Design review of the part built by this model. Coordinates are the model's own, in mm. A direction names the side the tool comes from. Give positions to 0.01 mm unless a question says otherwise; leave off trailing zeros. Loops run counter-clockwise (first coordinate to the right, second up) from the corner with the lowest first, then second, coordinate; pieces in that order, holes last.
from build123d import *

# Parameters (mm, degrees)
PAD002_DEPTH    = 10
SKETCH005_R     = 1.5
SKETCH005_W     = 170
SKETCH005_H     = 57.5
POCKET002_DEPTH = 11
PAD003_DEPTH    = 10
PAD004_DEPTH    = 10
POCKET003_DEPTH = 3
SKETCH009_W     = 103.713421
SKETCH009_H     = 5
POCKET004_DEPTH = 10
SKETCH010_W     = 109.037471
SKETCH010_H     = 5
POCKET005_DEPTH = 10
SKETCH011_R     = 1.5
POCKET006_DEPTH = 5
SKETCH012_R     = 3
POCKET007_DEPTH = 3


with BuildPart() as part:
    # Sketch004 → Pad002 (new body)
    with BuildSketch(Plane.XY.offset(-30)):
        Polygon((10, -50), (0, -50), (0, -40), (10, -40), (10, -15), (190, -15), (190, -40), (200, -40), (200, -50), (190, -50), (190, -120), (200, -120), (200, -130), (190, -130), (190, -150), (10, -150), (10, -130.022141), (0, -130.022141), (0, -120.229309), (10, -120.229309), align=None)
    extrude(amount=PAD002_DEPTH)

    # Sketch005 → Pocket002 (cut)
    with BuildSketch(Plane.XY.offset(-20)):
        with Locations((65, -82.5)):
            Circle(SKETCH005_R)
        with Locations((135, -82.5)):
            Circle(SKETCH005_R)
        with Locations((100, -48.75)):
            Rectangle(SKETCH005_W, SKETCH005_H)
        with Locations((100, -116.25)):
            Rectangle(SKETCH005_W, SKETCH005_H)
    extrude(amount=-POCKET002_DEPTH, mode=Mode.SUBTRACT)

    # Sketch006 → Pad003 (new body)
    with BuildSketch(Plane.XY.offset(-20)):
        Polygon((15.544486, -15), (9.942795, -23.283783), (183.213308, -150), (189.107285, -141.92157), align=None)
    extrude(amount=-PAD003_DEPTH)

    # Sketch007 → Pad004 (new body)
    with BuildSketch(Plane.XY.offset(-20)):
        Polygon((16.445199, -150), (10.823256, -141.729948), (182.344322, -15), (188.253036, -23.067658), align=None)
    extrude(amount=-PAD004_DEPTH)

    # Sketch008 → Pocket003 (cut)
    with BuildSketch(Plane(origin=(0, 0, -30), x_dir=(1, 0, 0), z_dir=(0, 0, -1))):
        Polygon((66.72504, 85.516563), (63.260938, 85.516563), (61.528887, 82.516563), (63.260938, 79.516563), (66.72504, 79.516563), (68.457091, 82.516563), align=None)
        Polygon((136.743449, 85.423233), (133.279347, 85.423233), (131.547296, 82.423233), (133.279347, 79.423233), (136.743449, 79.423233), (138.4755, 82.423233), align=None)
    extrude(amount=-POCKET003_DEPTH, mode=Mode.SUBTRACT)

    # Sketch009 → Pocket004 (cut)
    with BuildSketch(Plane(origin=(0, 0, -30), x_dir=(0, -1, 0), z_dir=(-1, 0, 0))):
        with Locations((85.35563, 2.5)):
            Rectangle(SKETCH009_W, SKETCH009_H)
    extrude(amount=-POCKET004_DEPTH, mode=Mode.SUBTRACT)

    # Sketch010 → Pocket005 (cut)
    with BuildSketch(Plane(origin=(200, 0, -30), x_dir=(0, 1, 0), z_dir=(1, 0, 0))):
        with Locations((-86.823625, 2.5)):
            Rectangle(SKETCH010_W, SKETCH010_H)
    extrude(amount=-POCKET005_DEPTH, mode=Mode.SUBTRACT)

    # Sketch011 → Pocket006 (cut)
    with BuildSketch(Plane.XY.offset(-20)):
        with Locations((5.036074, -44.974274)):
            Circle(SKETCH011_R)
        with Locations((4.981705, -125.071396)):
            Circle(SKETCH011_R)
        with Locations((194.832825, -45.021729)):
            Circle(SKETCH011_R)
        with Locations((194.878098, -125.009697)):
            Circle(SKETCH011_R)
    extrude(amount=-POCKET006_DEPTH, mode=Mode.SUBTRACT)

    # Sketch012 → Pocket007 (cut)
    with BuildSketch(Plane.XY.offset(-20)):
        with Locations((5.016462, -44.97184)):
            Circle(SKETCH012_R)
        with Locations((4.972344, -125.06855)):
            Circle(SKETCH012_R)
        with Locations((194.878128, -125.061401)):
            Circle(SKETCH012_R)
        with Locations((194.862854, -45.015846)):
            Circle(SKETCH012_R)
    extrude(amount=-POCKET007_DEPTH, mode=Mode.SUBTRACT)


solid = part.part
Q1. Draft analysis for pull direction Y (two halves, no side actions). For faces 6 (the face through (136.943, -48.546, -24.93)), 7 (the face through (10, -19, -25)), 8 (the face through (195, -130, -23)), state which applies: pulls with the +Y half, pulls with the -Y half, needs draft (parallel to the pull), parting line crosses it, or undercut.
Results:
face 6: undercut
face 7: needs draft
face 8: pulls with the -Y half
Q2. Take a section at D-D (y = -38). Give the boundary of the cut face in (x, z), plus the area to 3 significant figures.
Results:
outline: (10, -30) - (15, -30) - (15, -20) - (10, -20) - close; (30.07, -30) - (47, -30) - (47, -20) - (30.07, -20) - close; (151.22, -30) - (168.04, -30) - (168.04, -20) - (151.22, -20) - close; (185, -30) - (190, -30) - (190, -20) - (185, -20) - close
area: 438 mm2
Q3. Take a section at C-C (x = 57). Give the boundary of the cut face in (y, z).
Results:
outline: (-150, -30) - (-145, -30) - (-145, -20) - (-150, -20) - close; (-120.04, -30) - (-107.61, -30) - (-107.61, -20) - (-120.04, -20) - close; (-87.5, -30) - (-77.5, -30) - (-77.5, -20) - (-87.5, -20) - close; (-57.7, -30) - (-45.32, -30) - (-45.32, -20) - (-57.7, -20) - close; (-20, -30) - (-15, -30) - (-15, -20) - (-20, -20) - close
Q4. Take a section at A-A (y = -74). Give the boundary of the cut face in (x, z), plus the area to 3 significant figures.
Results:
outline: (10, -30) - (15, -30) - (15, -20) - (10, -20) - close; (79.29, -30) - (96.23, -30) - (96.23, -20) - (79.29, -20) - close; (102.49, -30) - (119.31, -30) - (119.31, -20) - (102.49, -20) - close; (185, -30) - (190, -30) - (190, -20) - (185, -20) - close
area: 438 mm2
Q5. Insertion check: pin 1 (2.5 mm diameter, centred on x = 5.04, y = -44.97, fed in from +Z); pin 2 (1.5 mm diameter, centred on x = 195.5, z = -23, fed in from -Y); pin 3 (3 mm diameter, centred on y = -98.5, z = -27, fed in from +X); pin 4 (3 mm diameter, centred on x = 6, y = -44, fed in from +Z). Each pin has a flat end and moves straight along its axis. Give the tip position at first contact, or say it passes through.
Results:
pin 1: passes through
pin 2: stops at y = -130
pin 3: stops at x = 190
pin 4: stops at z = -23
Q6. Tool access review of faces 1 (the face through (5, -50, -23)), 2 (the face through (195, -40, -23)), 3 (the face through (49, -77.5, -25)), 4 (the face through (5, -130.022, -23)), 5 (the face through (196.2, -44, -25)): name each direction out of +Z, -Z, +X, -X, +Y, -Y from which nothing blocks a thin tool from reaching the whole face with its end or side.
Results:
face 1: +Z, -Z, -X
face 2: +Z, -Z, +X, +Y
face 3: +Z, -Z
face 4: +Z, -Z, -X, -Y
face 5: -Z, +X, +Y, -Y
Q7. Wall thickness on line 1 (X direction, y = -82.5, z = -25); line 2 (Y direction, x = 21.5, z = -27); line 3 (Y direction, x = 34, z = -28.25): over which ranges is each line inside the solid? List them lowest first.
Results:
line 1: x = 10 to 63.5, 66.5 to 133.5, 136.5 to 190
line 2: y = -150 to -133.84, -87.5 to -77.5, -31.74 to -15
line 3: y = -150 to -145, -137.03 to -124.61, -87.5 to -77.5, -40.88 to -28.5, -20 to -15
Q8. Take a section at B-B (x = 19). Give the boundary of the cut face in (y, z).
Results:
outline: (-150, -30) - (-135.69, -30) - (-135.69, -20) - (-150, -20) - close; (-87.5, -30) - (-77.5, -30) - (-77.5, -20) - (-87.5, -20) - close; (-29.91, -30) - (-15, -30) - (-15, -20) - (-29.91, -20) - close
